Build history of the part. All positions in model axes, mm. Face numbers are marked on the shaded views. A direction names the side the tool comes from. Give positions to 0.01 mm unless a question says otherwise; leave off trailing zeros. Loops run counter-clockwise (first coordinate to the right, second up) from the corner with the lowest first, then second, coordinate; pieces in that order, holes last. Notation, with made-up numbers: (16.5, 66.25) -> (58.5, 66.25) arc R15 cw to (58.5, 74.25) -> close; hole circle Ø5 at (29, -27). An arc over 180 degrees is marked (long way). Answer as a JSON object with one key per item and string values. Group by question number.
Q1. Tool access for the marked faces 4 and 5: list every direction of +Z, -Z, +X, -X, +Y, -Y with a clear straight run to the whole face (end or side of a thin tool).
Q2. Two-plate mould, pull along X, no slides. Class the marked faces 1, 2 and 3: pulls with the +X half, pulls with the -X half, needs draft (parallel to the pull), parting line crosses it, or undercut.
Q3. Band-saw the part on B-B, the plane z = 17. Count the separate pieces of the cut face and the enclosed holes in it, plus the area to 3 significant figures.
Q4. Band-saw the part on C-C, the plane x = 36. Write the cut outline in (y, z) (1 decimal).
Q5. Wall check: probe 1 along Y at (x, z) = (152, 75); probe 2 along X at (y, z) = (0, 67.25); probe 3 along X at (y, z) = (164.5, 30.5) (1 decimal). Give the ranges that are in metal, low to high. Write a range as from..to.
Q6. Band-saw the part on A-A, the plane y = -101.6. Write the cut outline in (x, z) (1 decimal), plus the area to 3 significant figures.
Q7. Band-saw the part on D-D, the plane y = 101. Write the cut outline in (x, z) (1 decimal).
Q8. Drop flat-ended pins along their axis: pin 1 (16.5 mm diameter, centred on x = 152.4, y = 0, fed in from +Z); pin 2 (14.5 mm diameter, centred on x = 152.4, y = 114.3, fed in from -Z) (3 decimals). Give the stop position or say it passes through.
from build123d import *

# Parameters (mm, degrees)
F0_W     = 406.4
F0_H     = 406.4
F1_DEPTH = 76.2
F2_R     = 12.7
F3_R     = 4.7625
F4_DEPTH = 25.4
F5_R     = 6.35
F6_DEPTH = 25.4
F8_DEPTH = 73.025


with BuildPart() as f1:
    # F0 (on Top) → F1 (new body)
    with BuildSketch(Plane.XY):
        Rectangle(F0_W, F0_H)
    extrude(amount=F1_DEPTH)

    # F2
    f2_edges = [f1.edges().sort_by_distance(p)[0] for p in [
        (203.2, -203.2, 38.1),
        (-203.2, -203.2, 38.1),
        (203.2, 203.2, 38.1),
        (-203.2, 203.2, 38.1),
    ]]
    fillet(f2_edges, radius=F2_R)

    # F3 (on face) → F4 (cut)
    with BuildSketch(Plane.YZ.offset(203.2)):
        with Locations((-101.6, 31.75)):
            Circle(F3_R)
    extrude(amount=-F4_DEPTH, mode=Mode.SUBTRACT)

    # F5 (on face) → F6 (cut)
    with BuildSketch(Plane.XY.offset(76.2)):
        with Locations((152.4, -114.3)):
            Circle(F5_R)
        with Locations((152.4, 0)):
            Circle(F5_R)
        with Locations((152.4, 114.3)):
            Circle(F5_R)
    extrude(amount=-F6_DEPTH, mode=Mode.SUBTRACT)

    # F7 (on face) → F8 (cut)
    with BuildSketch(Plane(origin=(0, 0, 0), x_dir=(1, 0, 0), z_dir=(0, 0, -1))):
        Polygon((200.025, 1.5875), (200.025, 149.225), (151.4700640303, 149.225), (3.8325640303, 1.5875), align=None)
        Polygon((1.5875, 3.8325640303), (149.225, 151.4700640303), (149.225, 200.025), (1.5875, 200.025), align=None)
        Polygon((-1.5875, 200.025), (-149.225, 200.025), (-149.225, 151.4700640303), (-1.5875, 3.8325640303), align=None)
        Polygon((-3.8325640303, 1.5875), (-151.4700640303, 149.225), (-200.025, 149.225), (-200.025, 1.5875), align=None)
        Polygon((-200.025, -1.5875), (-200.025, -149.225), (-151.4700640303, -149.225), (-3.8325640303, -1.5875), align=None)
        Polygon((-1.5875, -3.8325640303), (-149.225, -151.4700640303), (-149.225, -200.025), (-1.5875, -200.025), align=None)
        Polygon((1.5875, -200.025), (149.225, -200.025), (149.225, -151.4700640303), (1.5875, -3.8325640303), align=None)
        Polygon((3.8325640303, -1.5875), (151.4700640303, -149.225), (200.025, -149.225), (200.025, -1.5875), align=None)
    extrude(amount=-F8_DEPTH, mode=Mode.SUBTRACT)


solid = f1.part
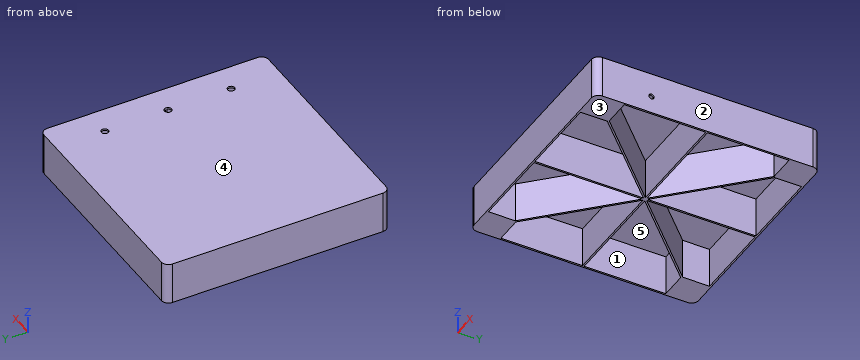
Worked answers:
{
 "1": {"face 4": "+Z, +X, -X, +Y, -Y", "face 5": "-Z"},
 "2": {"face 1": "undercut", "face 2": "pulls with the +X half", "face 3": "needs draft"},
 "3": {"separate pieces": "1", "enclosed holes": "8", "area": "20,500 mm2"},
 "4": {"outline": "(-203.2, 0) -> (-200, 0) -> (-200, 73) -> (-38.2, 73) -> (-38.2, 0) -> (-33.8, 0) -> (-33.8, 73) -> (-1.6, 73) -> (-1.6, 0) -> (1.6, 0) -> (1.6, 73) -> (33.8, 73) -> (33.8, 0) -> (38.2, 0) -> (38.2, 73) -> (200, 73) -> (200, 0) -> (203.2, 0) -> (203.2, 76.2) -> (-203.2, 76.2) -> close"},
 "5": {"probe 1": "-203.2..-120.64, -107.96..-6.34, 6.34..107.96, 120.64..203.2", "probe 2": "-203.2..146.05, 158.75..203.2", "probe 3": "-203.2..-149.2, -1.6..1.6, 149.2..203.2"},
 "6": {"outline": "(-203.2, 0) -> (-200, 0) -> (-200, 73) -> (-103.8, 73) -> (-103.8, 0) -> (-99.4, 0) -> (-99.4, 73) -> (-1.6, 73) -> (-1.6, 0) -> (1.6, 0) -> (1.6, 73) -> (99.4, 73) -> (99.4, 0) -> (103.8, 0) -> (103.8, 73) -> (200, 73) -> (200, 36.5) -> (203.2, 36.5) -> (203.2, 76.2) -> (-203.2, 76.2) -> close; (200, 0) -> (203.2, 0) -> (203.2, 27) -> (200, 27) -> close", "area": "2,610 mm2"},
 "7": {"outline": "(-203.2, 0) -> (-200, 0) -> (-200, 73) -> (-103.2, 73) -> (-103.2, 0) -> (-98.8, 0) -> (-98.8, 73) -> (-1.6, 73) -> (-1.6, 0) -> (1.6, 0) -> (1.6, 73) -> (98.8, 73) -> (98.8, 0) -> (103.2, 0) -> (103.2, 73) -> (200, 73) -> (200, 0) -> (203.2, 0) -> (203.2, 76.2) -> (-203.2, 76.2) -> close"},
 "8": {"pin 1": "z = 76.2", "pin 2": "z = 73.025"}
}
